from build123d import *

# Parameters (mm, degrees)
BOSS_EXTRUDE1_DEPTH      = 10
BOSS_EXTRUDE1_DEPTH_BACK = 7.437731252
BOSS_EXTRUDE2_DEPTH      = 50
FILLET7_R                = 10
FILLET9_R                = 10
FILLET10_R               = 10
CUT_EXTRUDE1_DEPTH       = 30
CUT_EXTRUDE1_DEPTH_BACK  = 30
SKETCH5_R                = 2.05
CUT_EXTRUDE2_START       = -17.437731252
CUT_EXTRUDE2_DEPTH       = 17.437731252


# Read off the part's stored shape, not the designer's step: Cut-Extrude2
with BuildPart() as part:
    # Sketch2 → Boss-Extrude1 (new, two sides: drawn at the far end of the back side and taken through both)
    with BuildSketch(Plane(origin=(0, 0, 0), x_dir=(0, 0, -1), z_dir=(1, 0, 0)).offset(-BOSS_EXTRUDE1_DEPTH_BACK)):
        with BuildLine():
            Line((100, 0), (130.792862778, -114.920528399))
            ThreePointArc((130.792862778, -114.920528399), (127.318193667, -142.802769687), (105.386466731, -160.366711677))
            Line((105.386466731, -160.366711677), (95.023521596, -163.453246629))
            ThreePointArc((95.023521596, -163.453246629), (65.300089376, -159.771732448), (47.8454422, -135.433054144))
            Line((47.8454422, -135.433054144), (35, -75))
            Line((35, -75), (-35, -75))
            Line((-35, -75), (-47.8454422, -135.433054144))
            ThreePointArc((-47.8454422, -135.433054144), (-65.300089376, -159.771732448), (-95.023521596, -163.453246629))
            Line((-95.023521596, -163.453246629), (-105.386466731, -160.366711677))
            ThreePointArc((-105.386466731, -160.366711677), (-127.318193667, -142.802769687), (-130.792862778, -114.920528399))
            Line((-130.792862778, -114.920528399), (-100, 0))
            Line((-100, 0), (-35, 0))
            Line((-35, 0), (35, 0))
            Line((35, 0), (100, 0))
        make_face()
    extrude(amount=BOSS_EXTRUDE1_DEPTH + BOSS_EXTRUDE1_DEPTH_BACK)

    # Sketch3 → Boss-Extrude2 (add)
    with BuildSketch(Plane(origin=(10, 0, 0), x_dir=(0, 0, -1), z_dir=(1, 0, 0))):
        with BuildLine():
            Line((100, 0), (130.792862778, -114.920528399))
            ThreePointArc((130.792862778, -114.920528399), (127.318193667, -142.802769687), (105.386466731, -160.366711677))
            Line((105.386466731, -160.366711677), (95.023521596, -163.453246629))
            ThreePointArc((95.023521596, -163.453246629), (65.300089376, -159.771732448), (47.8454422, -135.433054144))
            Line((47.8454422, -135.433054144), (35, -75))
            Line((35, -75), (70, -75))
            ThreePointArc((70, -75), (91.213203436, -66.213203436), (100, -45))
            Line((100, -45), (100, 0))
        make_face()
        with BuildLine():
            Line((-35, -75), (-47.8454422, -135.433054144))
            ThreePointArc((-47.8454422, -135.433054144), (-65.300089376, -159.771732448), (-95.023521596, -163.453246629))
            Line((-95.023521596, -163.453246629), (-105.386466731, -160.366711677))
            ThreePointArc((-105.386466731, -160.366711677), (-127.318193667, -142.802769687), (-130.792862778, -114.920528399))
            Line((-130.792862778, -114.920528399), (-100, 0))
            Line((-100, 0), (-100, -45))
            ThreePointArc((-100, -45), (-91.213203436, -66.213203436), (-70, -75))
            Line((-70, -75), (-35, -75))
        make_face()
    extrude(amount=BOSS_EXTRUDE2_DEPTH)

    # Fillet7
    fillet7_edges = [part.edges().sort_by_distance(p)[0] for p in [
        (60, -57.4602642, 115.396431389),
        (60, -142.802769687, 127.318193667),
        (60, -161.909979153, 100.204994164),
        (60, -159.771732448, 65.300089376),
        (60, -105.216527072, 41.4227211),
    ]]
    fillet(fillet7_edges, radius=FILLET7_R)

    # Fillet9
    fillet9_edges = [part.edges().sort_by_distance(p)[0] for p in [
        (60, -105.216527072, -41.4227211),
        (60, -159.771732448, -65.300089376),
        (60, -161.909979153, -100.204994164),
        (60, -142.802769687, -127.318193667),
        (60, -57.4602642, -115.396431389),
    ]]
    fillet(fillet9_edges, radius=FILLET9_R)

    # Fillet10
    fillet10_edges = [part.edges().sort_by_distance(p)[0] for p in [
        (-7.437731252, -57.4602642, 115.396431389),
        (-7.437731252, -142.802769687, 127.318193667),
        (-7.437731252, -161.909979153, 100.204994164),
        (-7.437731252, -159.771732448, 65.300089376),
        (-7.437731252, -105.216527072, 41.4227211),
        (-7.437731252, -105.216527072, -41.4227211),
        (-7.437731252, -159.771732448, -65.300089376),
        (-7.437731252, -161.909979153, -100.204994164),
        (-7.437731252, -142.802769687, -127.318193667),
        (-7.437731252, -57.4602642, -115.396431389),
    ]]
    fillet(fillet10_edges, radius=FILLET10_R)

    # Sketch5 → Cut-Extrude1 (cut, two sides: drawn at the far end of the back side and taken through both)
    with BuildSketch(Plane(origin=(10, 0, 0), x_dir=(0, 0, -1), z_dir=(1, 0, 0)).offset(-CUT_EXTRUDE1_DEPTH_BACK)):
        with Locations(Location((45, -62.5, 0), (0, 0, 180))):
            Circle(SKETCH5_R)
        with Locations(Location((-45, -62.5, 0), (0, 0, 180))):
            Circle(SKETCH5_R)
        with Locations(Location((-45, -22.5, 0), (0, 0, 180))):
            Circle(SKETCH5_R)
        with Locations(Location((45, -22.5, 0), (0, 0, 180))):
            Circle(SKETCH5_R)
    extrude(amount=CUT_EXTRUDE1_DEPTH + CUT_EXTRUDE1_DEPTH_BACK, mode=Mode.SUBTRACT)

    # Cut-Extrude2 outline → Cut-Extrude2 (cut)
    with BuildSketch(Plane(origin=(10, 0, 0), x_dir=(0, 0, -1), z_dir=(1, 0, 0)).offset(CUT_EXTRUDE2_START)):
        with BuildLine():
            ThreePointArc((70, -75), (91.213203436, -66.213203436), (100, -45))
            Line((100, -45), (100, -38.637033052))
            Line((100, -38.637033052), (70, -38.637033052))
            Line((70, -38.637033052), (70, -75))
        make_face()
        with BuildLine():
            ThreePointArc((-100, -45.17228394), (-91.263664233, -66.263664233), (-70.17228394, -75))
            Line((-70.17228394, -75), (-70, -75))
            Line((-70, -75), (-70, -38.637033052))
            Line((-70, -38.637033052), (-100, -38.637033052))
            Line((-100, -38.637033052), (-100, -45.17228394))
        make_face()
    extrude(amount=CUT_EXTRUDE2_DEPTH, mode=Mode.SUBTRACT)


solid = part.part
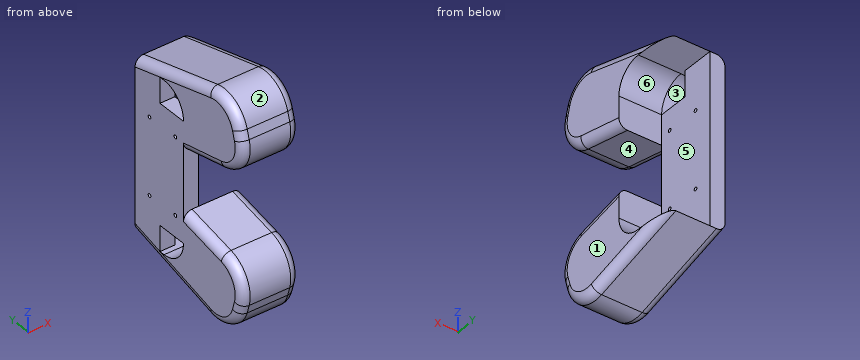
Source: CAD feature listing. Evaluate the final solid. Frame: model axes, mm. Face numbers are marked on the shaded views. A direction names the side the tool comes from. Give positions to 0.01 mm unless a question says otherwise; leave off trailing zeros. Order: outer loops, then holes, each group sorted by start corner. A loop starts at its lowest first (then second) coordinate and runs counter-clockwise, first axis right, second up. Notation, with made-up numbers: (69, 11) -> (80, 11) arc R9 cw to (80, 26) -> close; hole circle Ø2 at (81.25, 84). An arc over 180 degrees is marked (long way). Write item = value, one per line.
Item 1: Set-up query: the marked faces 4, 5 and 6. Return all of +Z, -Z, +X, -X, +Y, -Y with unobstructed straight access to the full face (end or side cutting, diameter ignored); none if empty.
Check result:
face_4 = +X, -X, -Y
face_5 = +X, +Y
face_6 = +X, -X, +Y
Item 2: Contact query for flat-ended pins moving along their axis: pin 1 (5 mm diameter, centred on x = 0, y = -52.5, fed in from +Z); pin 2 (22.5 mm diameter, centred on x = 42.5, y = -28, fed in from -Z); pin 3 (17.5 mm diameter, centred on x = 38, z = 50, fed in from +Y); pin 4 (3.5 mm diameter, centred on y = -62.5, z = 45, fed in from -X). Output: stop coordinate, or through.
Check result:
pin_1 = 114.56
pin_2 = -110.52
pin_3 = -75
pin_4 = through
Item 3: Section query C-C (y = -69). State how many separate pieces and enclosed holes the cut face has, then the cut area to 3 significant figures.
Check result:
separate_pieces = 3
enclosed_holes = 0
area = 6,460 mm²
Item 4: Ray query, probe 1 along Y at (x, z) = (1, 11); probe 2 along Z at (x, y) = (27, -82); probe 3 along Z at (x, y) = (42.5, -39). Return the intervals inside material, ascending.
Check result:
probe_1 = -75 to 0
probe_2 = -121.97 to -36.49, 36.49 to 121.97
probe_3 = -110.45 to -100, 100 to 110.45
Item 5: Section query A-A (x = 34). Output: boundary loops of the cut face in (y, z), then the cut area to 3 significant figures.
Check result:
outline = (-163.45, -95.02) -> (-160.37, -105.39) arc R37.34 ccw to (-114.92, -130.79) -> (0, -100) -> (-45, -100) arc R30 cw to (-75, -70) -> (-75, -35) -> (-135.43, -47.85) arc R37.34 ccw to start; (-163.45, 95.02) arc R37.34 ccw to (-135.43, 47.85) -> (-75, 35) -> (-75, 70) arc R30 cw to (-45, 100) -> (0, 100) -> (-114.92, 130.79) arc R37.34 ccw to (-160.37, 105.39) -> close
area = 15,900 mm²
Item 6: Mould query, pull axis Y, two halves, no side actions, for the marked faces 1, 2 and 3. Classes: +Y half, -Y half, draft (parallel to the pull), parting line (faces both ways), or undercut.
Check result:
face_1 = draft
face_2 = parting line
face_3 = undercut
Item 7: Section query B-B (z = -24.5). Output: boundary loops of the cut face in (x, y), then the cut area to 3 significant figures.
Check result:
outline = (-7.44, -75) -> (10, -75) -> (10, 0) -> (-7.44, 0) -> close
area = 1,310 mm²
